Drawing for the job (mm, zero at the part's lowest x, y, z). Coordinates: 2 decimals unless noted, no trailing zeros. Write each loop counter-clockwise with the first axis right and the second up, starting at its lowest first coordinate (ties: lowest second). Pieces come first, ordered by that corner, then holes. Notation, with made-up numbers: (15, -10.75) -> (56, -10.75) arc R25 ccw to (56, 17.25) -> close; hole circle Ø11 at (80, 89.5). An arc over 180 degrees is marked (long way). Write item = value, one per line. Start each with the question number.
Q1. Band-saw the part on C-C, the plane x = 262. List the corners of the cut face in (y, z).
Q2. Probe line 1 (Z direction, x = 242, y = 4); line 2 (X direction, y = 0.5, z = 50.5); line 3 (X direction, y = 4, z = 22.5). List the from-to ranges inside material, lowest first.
Q3. Band-saw the part on B-B, the plane z = 57. List the corners of the cut face in (x, y), plus the area to 3 significant figures.
Q4. Band-saw the part on A-A, the plane y = 5. List the corners of the cut face in (x, z), plus the area to 3 significant figures.
Q5. Pin check, flat tips, straight feed: P1, Ø1.9, axis at x = 13.5, y = 2.5, coming from the -Z side; P2, Ø2, axis at y = 4.5, z = 49, coming from the +X side; P3, Ø1, axis at y = 4, z = 66.5, coming from the +X side. Stop position of each tip, or through.
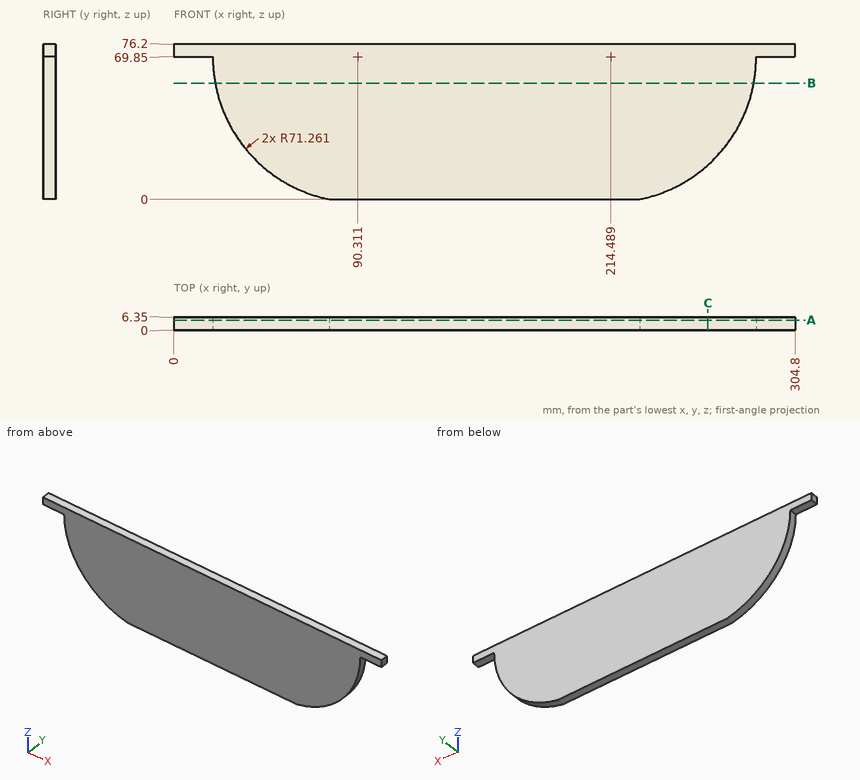
Ans:
q1.outline = (0, 16.74) -> (6.35, 16.74) -> (6.35, 76.2) -> (0, 76.2) -> close
q2.line_1 = 4.11 to 76.2
q2.line_2 = 21.73 to 283.07
q2.line_3 = 37.06 to 267.74
q3.outline = (20.22, 0) -> (284.58, 0) -> (284.58, 6.35) -> (20.22, 6.35) -> close
q3.area = 1,680 mm2
q4.outline = (0, 69.85) -> (19.05, 69.85) arc R71.26 ccw to (76.2, 0) -> (228.6, 0) arc R71.26 ccw to (285.75, 69.85) -> (304.8, 69.85) -> (304.8, 76.2) -> (0, 76.2) -> close
q4.area = 18,600 mm2
q5.P1 = 69.85
q5.P2 = 282.93
q5.P3 = 285.69
